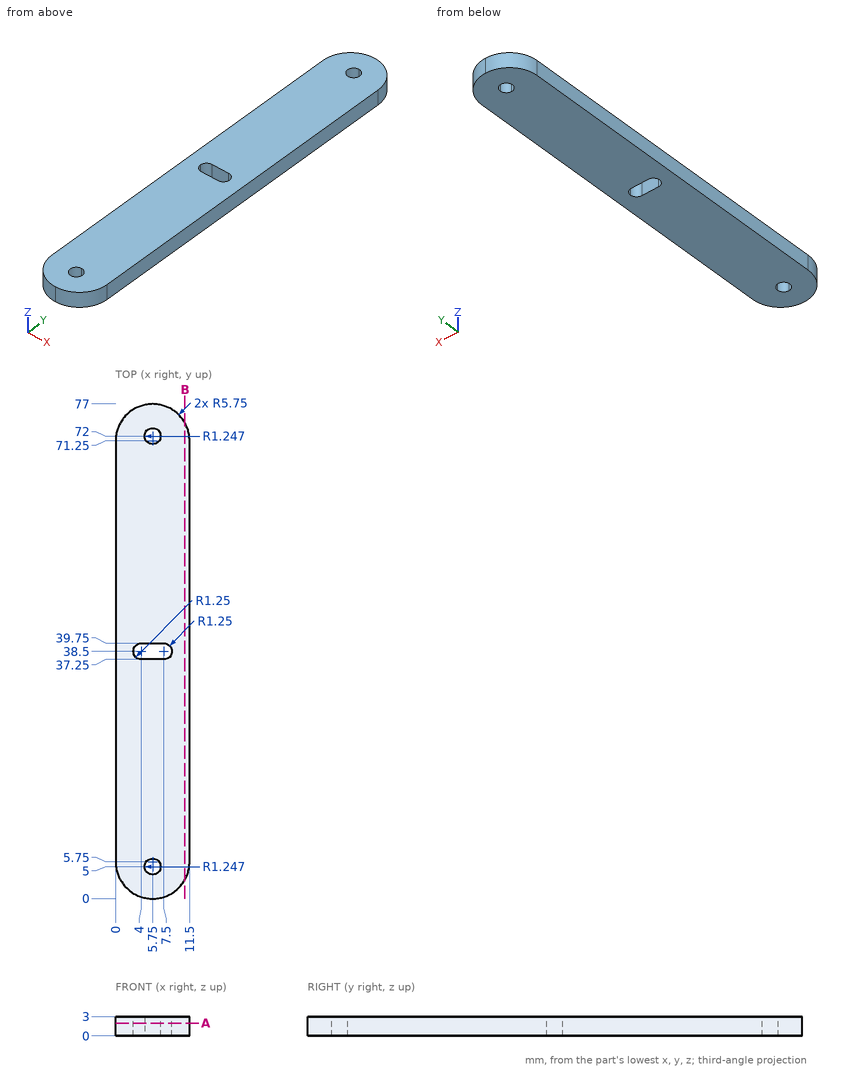
Here's the drawing with two shaded views (mm, measured from the low corner). I have some questions. Coordinates: 2 decimals unless noted, no trailing zeros. Order: outer loops, then holes, each group sorted by start corner. A loop starts at its lowest first (then second) coordinate and runs counter-clockwise, first axis right, second up. Notation, with made-up numbers: (52.25, 61) - (99.25, 61) arc R17 cw to (99.25, 93) - close; hole circle Ø2 at (0, 50). An arc over 180 degrees is marked (long way). Answer in a Markdown table with one row per item.
1. If I drill on line 1 along Y through (x, z) = (6.25, 0.5); line 2 along Y through (x, z) = (7.75, 1.9) (1 decimal); line 3 along Y through (x, z) = (7.5, 2.15), over which ranges is the centre line in solid material (lowest first)?
Reply:
| item | result |
|---|---|
| line 1 | y = 0.02 to 3.86, 6.14 to 37.25, 39.75 to 70.86, 73.14 to 76.98 |
| line 2 | y = 0.4 to 37.3, 39.7 to 76.6 |
| line 3 | y = 0.27 to 37.25, 39.75 to 76.73 |
2. Suppose I cut it at B-B (x = 10.75). Please give me the cut outline in (y, z).
Reply:
| item | result |
|---|---|
| outline | (2.91, 0) - (74.09, 0) - (74.09, 3) - (2.91, 3) - close |
3. Suppose I cut it at A-A (z = 2). Please give me the cut outline in (x, y), and give its area (3 significant figures).
Reply:
| item | result |
|---|---|
| outline | (0, 5.75) arc R5.75 ccw to (11.5, 5.75) - (11.5, 71.25) arc R5.75 ccw to (0, 71.25) - close; hole (4, 37.25) - (7.5, 37.25) arc R1.25 ccw to (8.75, 38.5) arc R1.25 ccw to (7.5, 39.75) - (4, 39.75) arc R1.25 ccw to start; hole (5.75, 3.75) arc R1.25 ccw to (7, 5) arc R1.25 ccw to (5.75, 6.25) arc R1.25 ccw to start; hole (5.75, 70.75) arc R1.25 ccw to (7, 72) arc R1.25 ccw to (5.75, 73.25) arc R1.25 ccw to start |
| area | 834 mm^2 |
